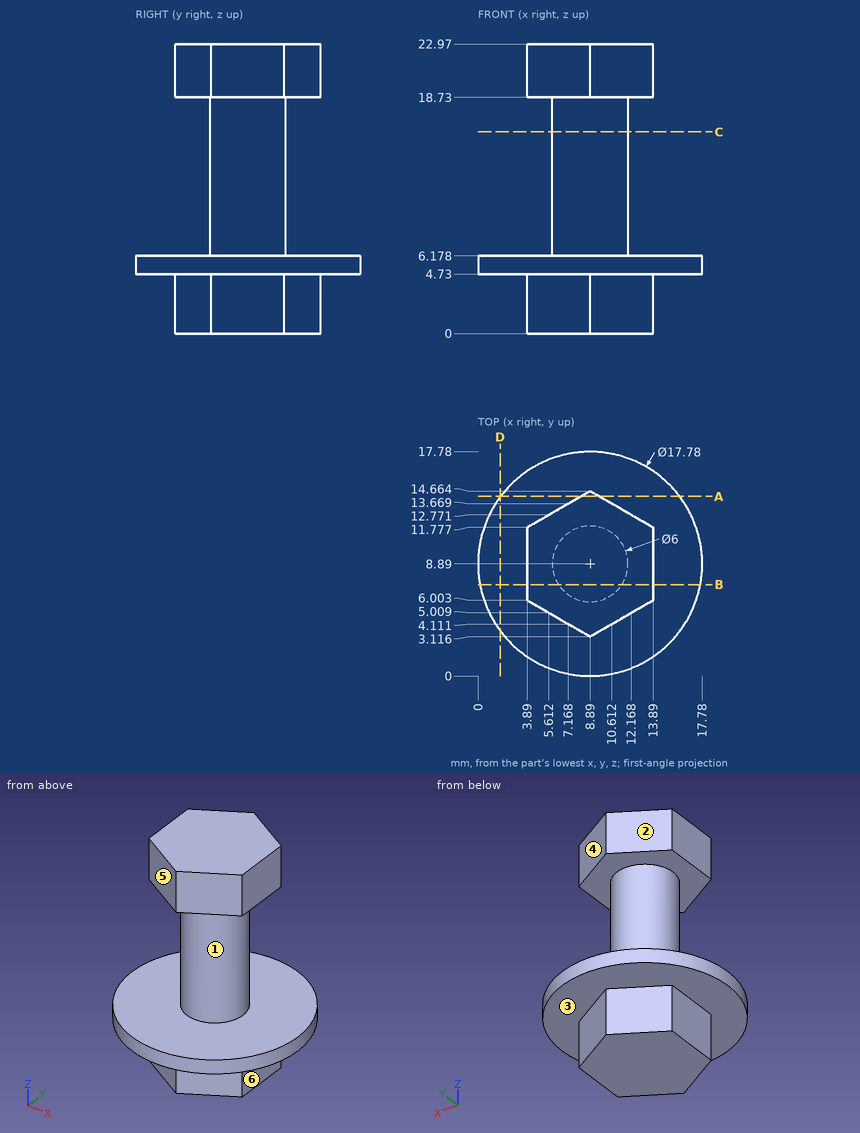
Check sheet for the drawn part. Datum: minimum x, y, z corner. Units: mm. A direction names the side the tool comes from. Round coordinates to 2 decimals unless told otherwise and drop trailing zeros. Loops run counter-clockwise (first coordinate to the right, second up) from the corner with the lowest first, then second, coordinate; pieces in that order, holes last. Notation, with made-up numbers: (-33, 18.5) -> (9, 18.5) arc R25 ccw to (9, 43.5) -> close; hole circle Ø1 at (-29, 34). An arc over 180 degrees is marked (long way). Put each result on its own line as item: value. Start each with the question number.
1. Access from +Z, -Z, +X, -X, +Y, -Y to the whole of each face (thin tool, end or side, straight path). Record for the marked faces 4, 5 and 6.
2. Section check B-B (y = 7.25). Enter the section's corners in (x, z).
3. Section check C-C (z = 16). Enter the section's corners in (x, y).
4. Section check D-D (x = 1.75). Enter the section's corners in (y, z).
5. Gauge pin test, flat ends, axial feed: pin 1 (5 mm diameter, centred on y = 15.5, z = 4, fed in from +X) (1 decimal); pin 2 (1.4 mm diameter, centred on y = 9.5, z = 3, fed in from +X); pin 3 (2 mm diameter, centred on y = 9, z = 8.5, fed in from -X); pin 4 (4 mm diameter, centred on x = 15, z = 16.5, fed in from +Y). Record the tip position at first contact, or that the pin passes through.
6. Section check A-A (y = 14.25). Enter the section's corners in (x, z).
7. Scan lines: probe 1 along Z at (x, y) = (10.75, 11.5); probe 2 along X at (y, z) = (11.5, 2.75); probe 3 along Z at (x, y) = (15.5, 4.5). Record each from-to range of solid material in increasing order.
8. Draft check along Z on the marked faces 1, 2 and 3. Enter one of: +Z half, -Z half, draft (parallel to the pull), parting line (faces both ways), or undercut.
Findings:
1. face 4: +Z, +X, +Y
1. face 5: +Z, -X, -Y
1. face 6: -Z, +X, +Y, -Y
2. outline: (0.15, 4.73) -> (3.89, 4.73) -> (3.89, 0) -> (13.89, 0) -> (13.89, 4.73) -> (17.63, 4.73) -> (17.63, 6.18) -> (11.4, 6.18) -> (11.4, 18.73) -> (13.89, 18.73) -> (13.89, 22.97) -> (3.89, 22.97) -> (3.89, 18.73) -> (6.38, 18.73) -> (6.38, 6.18) -> (0.15, 6.18) -> close
3. outline: circle Ø6 at (8.89, 8.89)
4. outline: (3.59, 4.73) -> (14.19, 4.73) -> (14.19, 6.18) -> (3.59, 6.18) -> close
5. pin 1: stops at x = 16.7
5. pin 2: stops at x = 13.89
5. pin 3: stops at x = 5.89
5. pin 4: passes through
6. outline: (1.8, 4.73) -> (8.17, 4.73) -> (8.17, 0) -> (9.61, 0) -> (9.61, 4.73) -> (15.98, 4.73) -> (15.98, 6.18) -> (1.8, 6.18) -> close; (8.17, 18.73) -> (9.61, 18.73) -> (9.61, 22.97) -> (8.17, 22.97) -> close
7. probe 1: z = 0 to 6.18, 18.73 to 22.97
7. probe 2: x = 3.89 to 13.89
7. probe 3: z = 4.73 to 6.18
8. face 1: undercut
8. face 2: draft
8. face 3: -Z half
